```python
from build123d import *

# Parameters (mm, degrees)
F0_R     = 8.875
F1_DEPTH = 2
F2_R     = 2.5
F3_DEPTH = 14
F5_DEPTH = 4


with BuildPart() as f1:
    # F0 (on Top) → F1 (new body)
    with BuildSketch(Plane.XY):
        Circle(F0_R)
    extrude(amount=F1_DEPTH)

    # F2 (on face) → F3 (join)
    with BuildSketch(Plane(origin=(0, 0, 0), x_dir=(1, 0, 0), z_dir=(0, 0, -1))):
        Circle(F2_R)
    extrude(amount=F3_DEPTH)

    # F4 (on face) → F5 (join)
    with BuildSketch(Plane.XY.offset(2)):
        Polygon((-4.041452, 0), (-2.020726, -3.5), (2.020726, -3.5), (4.041452, 0), (2.020726, 3.5), (-2.020726, 3.5), align=None)
    extrude(amount=F5_DEPTH)


solid = f1.part
```
Geometry check sheet. Reference: the model listing, model coordinates, mm. A direction names the side the tool comes from. Round coordinates to 2 decimals unless told otherwise and drop trailing zeros. Write each loop counter-clockwise with the first axis right and the second up, starting at its lowest first coordinate (ties: lowest second). Pieces come first, ordered by that corner, then holes. Notation, with made-up numbers: (-20.5, 48) - (25.5, 48) arc R21 cw to (25.5, 56) - close; hole circle Ø8 at (79.25, 48). An arc over 180 degrees is marked (long way). Write each question's results on one line, items separated by ' | '.
(1) Sectioned sample at B-B, the plane y = 0.5. Enter the section's corners in (x, z).
Computed:
outline: (-8.86, 0) - (-2.45, 0) - (-2.45, -14) - (2.45, -14) - (2.45, 0) - (8.86, 0) - (8.86, 2) - (3.75, 2) - (3.75, 6) - (-3.75, 6) - (-3.75, 2) - (-8.86, 2) - close
(2) Sectioned sample at A-A, the plane x = 0. Enter the section's corners in (y, z) (3 decimals), plus the area to 4 significant figures.
Computed:
outline: (-8.875, 0) - (-2.5, 0) - (-2.5, -14) - (2.5, -14) - (2.5, 0) - (8.875, 0) - (8.875, 2) - (3.5, 2) - (3.5, 6) - (-3.5, 6) - (-3.5, 2) - (-8.875, 2) - close | area: 133.5 mm^2
(3) Depth check by flat-ended pin: pin 1 Ø1 at (x, z) = (2.5, -10.5) entering from -Y; pin 2 Ø10 at (y, z) = (-5.5, 2) entering from -X; pin 3 Ø3 at (x, z) = (-5.5, -10.5) entering from +Y; pin 4 Ø1.2 at (x, z) = (1, 5) entering from +Y. Enter the tip coordinate at first touch or a pass-through.
Computed:
pin 1: stops at y = -1.5 | pin 2: stops at x = -8.86 | pin 3: passes through | pin 4: stops at y = 3.5
(4) Set-up check for faces 1 (the face through (0, -4, 2)), 2 (the face through (0, -3.5, 4)), 3 (the face through (3.045, 1.726, 3.972)), 4 (the face through (3, -1.8, 4)), 5 (the face through (2, -2, 0)): record each of +Z, -Z, +X, -X, +Y, -Y from which the full face is reachable in a straight line by a thin tool's end or side.
Computed:
face 1: +Z | face 2: +Z, +X, -X, -Y | face 3: +Z, +X, +Y | face 4: +Z, +X, -Y | face 5: -Z
(5) Thickness scan on probe 1 along Z at (x, y) = (-5.75, -2.5); probe 2 along Z at (x, y) = (-2.5, 0.5); probe 3 along Y at (x, z) = (0.5, -6.5). Record the ranges inside material, lowest first. Write a range as from..to.
Computed:
probe 1: z = 0..2 | probe 2: z = 0..6 | probe 3: y = -2.45..2.45
(6) Sectioned sample at D-D, the plane z = 4.5. Enter the section's corners in (x, y).
Computed:
outline: (-4.04, 0) - (-2.02, -3.5) - (2.02, -3.5) - (4.04, 0) - (2.02, 3.5) - (-2.02, 3.5) - close
(7) Sectioned sample at C-C, the plane z = -10. Enter the section's corners in (x, y).
Computed:
outline: circle Ø5 at (0, 0)
